The listing builds one solid part. Answer for the finished solid, in the listing's coordinates (mm). Face numbers are marked on the shaded views. A direction names the side the tool comes from. Give positions to 0.01 mm unless a question says otherwise; leave off trailing zeros. Loops run counter-clockwise (first coordinate to the right, second up) from the corner with the lowest first, then second, coordinate; pieces in that order, holes last.
Item 1: Consider line 1 along Y through (x, z) = (19.5, 14); line 2 along X through (y, z) = (-2.5, 61). Determine where each line is inside the solid, lowest interval first.
Item 2: Section A-A, the plane z = 94.5 is taken. Give the vertices of the cut face in (x, y), and give its area (3 significant figures).
Item 3: A tool of negligible diameter and unlimited length cuts with its end or side. For the marked faces 1 and 2, from which of +Z, -Z, +X, -X, +Y, -Y can it reach the whole face along a straight path? Write none if from no direction.
Item 4: Each of these flat-tipped pins is pushed along its axis until it touches: pin 1 Ø1 at (y, z) = (5, 19) entering from +X; pin 2 Ø4 at (x, z) = (6.5, 52) entering from +Y. Where does it stop, or does it pass through?
Item 5: Section B-B, the plane x = 5 is taken. Give the vertices of the cut face in (y, z).
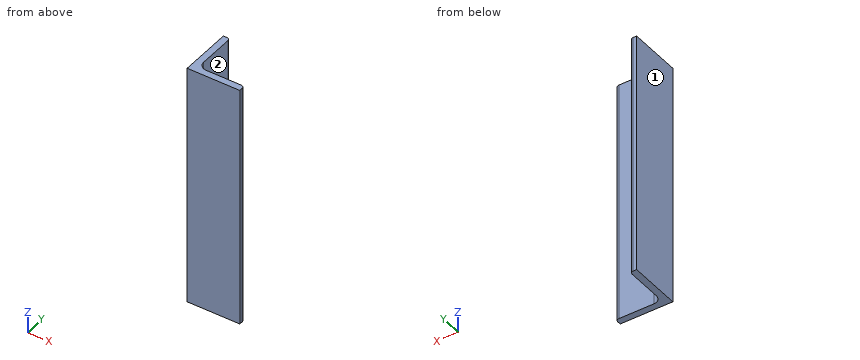
Autodesk Inventor part; units mm, degrees
ref_plane "Start Plane" through (0, 0, 0) normal (0, 0, 1) x (1, 0, 0)
ref_plane "End Plane" through (0, 0, 185) normal (0, 0, 1) x (1, 0, 0)
ref_plane "YZ Plane" through (0, 0, 0) normal (1, 0, 0) x (0, 1, 0)
ref_plane "Start Plane" through (0, 0, 0) normal (0, 0, 1) x (1, 0, 0)
ref_plane "End Plane" through (0, 0, 185) normal (0, 0, 1) x (1, 0, 0)
sketch "Sketch" plane through (0, 0, 0) normal (0, 0, 1) x (1, 0, 0)
  line L0 (-6.6013, -0.6013) -> (-6.6013, 25.9987)
  line L1 (-11.6013, 28.3987) -> (-9.0013, 28.3987)
  line L2 (-11.6013, -11.6013) -> (-11.6013, 28.3987)
  line L3 (-11.6013, -11.6013) -> (28.3987, -11.6013)
  line L4 (28.3987, -9.0013) -> (28.3987, -11.6013)
  line L5 (-0.6013, -6.6013) -> (25.9987, -6.6013)
  arc A0 (-6.6013, -0.6013) -> (-0.6013, -6.6013) centre (-0.6013, -0.6013) ccw
  arc A1 (-6.6013, 25.9987) -> (-9.0013, 28.3987) centre (-9.0013, 25.9987) ccw
  arc A2 (28.3987, -9.0013) -> (25.9987, -6.6013) centre (25.9987, -9.0013) ccw
  line L6 (0, 36.9952) -> (0, -19.7007) construction
  line L7 (-19.7007, 0) -> (36.9952, 0) construction
  point P0 (-6.6013, -6.6013)
  point P1 (-6.6013, 28.3987)
  point P2 (28.3987, -6.6013)
  dimension "d4" = 40
  dimension "d6" = 40
  dimension "d8" = 5
  dimension "d10" = 5
  dimension "d17" = 6
  dimension "d18" = 2.4
  dimension "d19" = 11.6013
  dimension "d20" = 11.6013
extrude "Body" add sketch "Sketch" along normal up to surface (185 mm away) from surface at 0
sketch "Sketch3" plane through (0, 0, 0) normal (0, 0, 1) x (1, 0, 0)
  line L0 (0, 0) -> (10, 0)
ref_plane "Work Plane10" through (0, 0, 0) normal (0, -1, 0) x (1, 0, 0)
sketch "Sketch4" plane through (0, 0, 0) normal (0, -1, 0) x (1, 0, 0)
  line L0 (-2, 0) -> (12, 0)
  line L1 (-2, 185) -> (12, 185)
  dimension "d24" = 185
equation "\"d4\" = b"
equation "\"d6\" = b"
equation "\"d17\" = R"
equation "\"d18\" = R1"
equation "\"d19\" = ex"
equation "\"d20\" = d19"
equation "\"d11\" = G_L"
equation "\"b\" = 40"
equation "\"ParT\" = 5"
equation "\"R\" = 6"
equation "\"R1\" = 2.4"
equation "\"G_L\" = d24"
equation "\"G_OFFSET_START\" = 0"
equation "\"G_OFFSET_END\" = 0"
equation "\"d22\" = G_OFFSET_END + B_L"
equation "\"B_L\" = 185"
properties part number "BS 4848 - 40x40x5-185" material "Steel, Mild"
Worked answers:
1. line 1: y = -11.6 to -6.6
1. line 2: x = -11.6 to -6.29
2. outline: (-11.6, -11.6) - (28.4, -11.6) - (28.4, -9) arc R2.4 ccw to (26, -6.6) - (-0.6, -6.6) arc R6 cw to (-6.6, -0.6) - (-6.6, 26) arc R2.4 ccw to (-9, 28.4) - (-11.6, 28.4) - close
2. area: 380 mm2
3. face 1: +Z, -Z, -X, +Y, -Y
3. face 2: +Z, -Z, +X, +Y
4. pin 1: stops at x = -6.6
4. pin 2: stops at y = -6.6
5. outline: (-11.6, 0) - (-6.6, 0) - (-6.6, 185) - (-11.6, 185) - close
